For this review, take the finished solid that the model builds, in its own axes (mm). Face numbers are marked on the shaded views. Round coordinates to 2 decimals unless told otherwise and drop trailing zeros. Order: outer loops, then holes, each group sorted by start corner. A loop starts at its lowest first (then second) coordinate and runs counter-clockwise, first axis right, second up. Notation, with made-up numbers: (-14.75, 6.25) - (26.25, 6.25) arc R15 ccw to (26.25, 33.25) - close; hole circle Ø1 at (39, 46). An arc over 180 degrees is marked (long way). One line per question, with ' | ' between items.
```python
from build123d import *

# Parameters (mm, degrees)
SKETCH1_W           = 3.125
SKETCH1_H           = 3.75
SKETCH2_R           = 5.25
SKETCH2_R_2         = 2.125
BOSS_EXTRUDE1_DEPTH = 16
SKETCH3_R           = 5.25
SKETCH3_R_2         = 3
CUT_EXTRUDE1_DEPTH  = 0.5


with BuildPart() as part:
    # Sketch1 → Revolve1 (revolve)
    with BuildSketch(Plane(origin=(0, 0, 0), x_dir=(1, 0, 0), z_dir=(0, 1, 0))):
        with Locations((3.6875, -1.875)):
            Rectangle(SKETCH1_W, SKETCH1_H)
    revolve(axis=Axis((0, 0, 0), (0, 0, 1)))

    # Sketch2 → Boss-Extrude1 (add)
    with BuildSketch(Plane.XY.offset(3.75)):
        Circle(SKETCH2_R)
        Circle(SKETCH2_R_2, mode=Mode.SUBTRACT)
    extrude(amount=BOSS_EXTRUDE1_DEPTH)

    # Sketch3 → Cut-Extrude1 (cut)
    with BuildSketch(Plane(origin=(0, 0, 0), x_dir=(-1, 0, 0), z_dir=(0, 0, -1))):
        Circle(SKETCH3_R)
        Circle(SKETCH3_R_2, mode=Mode.SUBTRACT)
    extrude(amount=-CUT_EXTRUDE1_DEPTH, mode=Mode.SUBTRACT)


solid = part.part
```
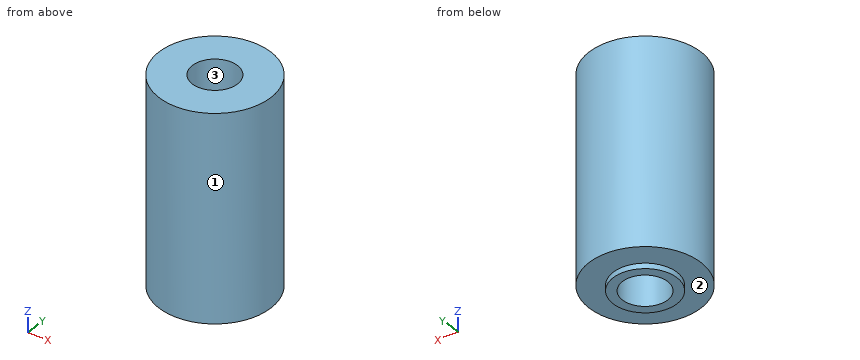
(1) Insertion check: pin 1 (1 mm diameter, centred on x = -2.5, z = 15.5, fed in from -Y); pin 2 (3 mm diameter, centred on x = 3, z = 5, fed in from -Y); pin 3 (3 mm diameter, centred on x = -1.5, z = 11.5, fed in from -Y). Each pin has a flat end and moves straight along its axis. Give the tip position at first contact, or say it passes through.
Output values:
pin 1: y = -4.85 | pin 2: y = -5.03 | pin 3: y = -5.25
(2) For probe 1 along Y at (x, z) = (0, 9) (3 decimals); probe 2 along Z at (x, y) = (-1.5, -4.5); probe 3 along X at (y, z) = (-1, 1.75) (3 decimals), list the stretches that pass through material, from the lowest coordinate up. Write a range as [from, to].
Output values:
probe 1: [-5.25, -2.125], [2.125, 5.25] | probe 2: [0.5, 19.75] | probe 3: [-5.154, -1.875], [1.875, 5.154]
(3) We need section C-C on z = 13. State the section outline as (x, y) points (3 decimals), plus the area to 3 significant figures.
Output values:
outline: circle Ø10.5 at (0, 0); hole circle Ø4.25 at (0, 0) | area: 72.4 mm^2
(4) We need section A-A on x = 0. State the section outline as (y, z) points (3 decimals).
Output values:
outline: (-5.25, 0.5) - (-3, 0.5) - (-3, 0) - (-2.125, 0) - (-2.125, 19.75) - (-5.25, 19.75) - close; (2.125, 0) - (3, 0) - (3, 0.5) - (5.25, 0.5) - (5.25, 19.75) - (2.125, 19.75) - close
(5) We need section D-D on y = 3.5. State the section outline as (x, z) points, plus the area to 3 significant figures.
Output values:
outline: (-3.91, 0.5) - (3.91, 0.5) - (3.91, 19.75) - (-3.91, 19.75) - close | area: 151 mm^2
(6) Mouldability with a two-part tool opening along X and no side actions: class the marked faces 1, 2 and 3 as released by +X, released by -X, zero draft, split by the parting line, or undercut.
Output values:
face 1: split by the parting line | face 2: zero draft | face 3: undercut
